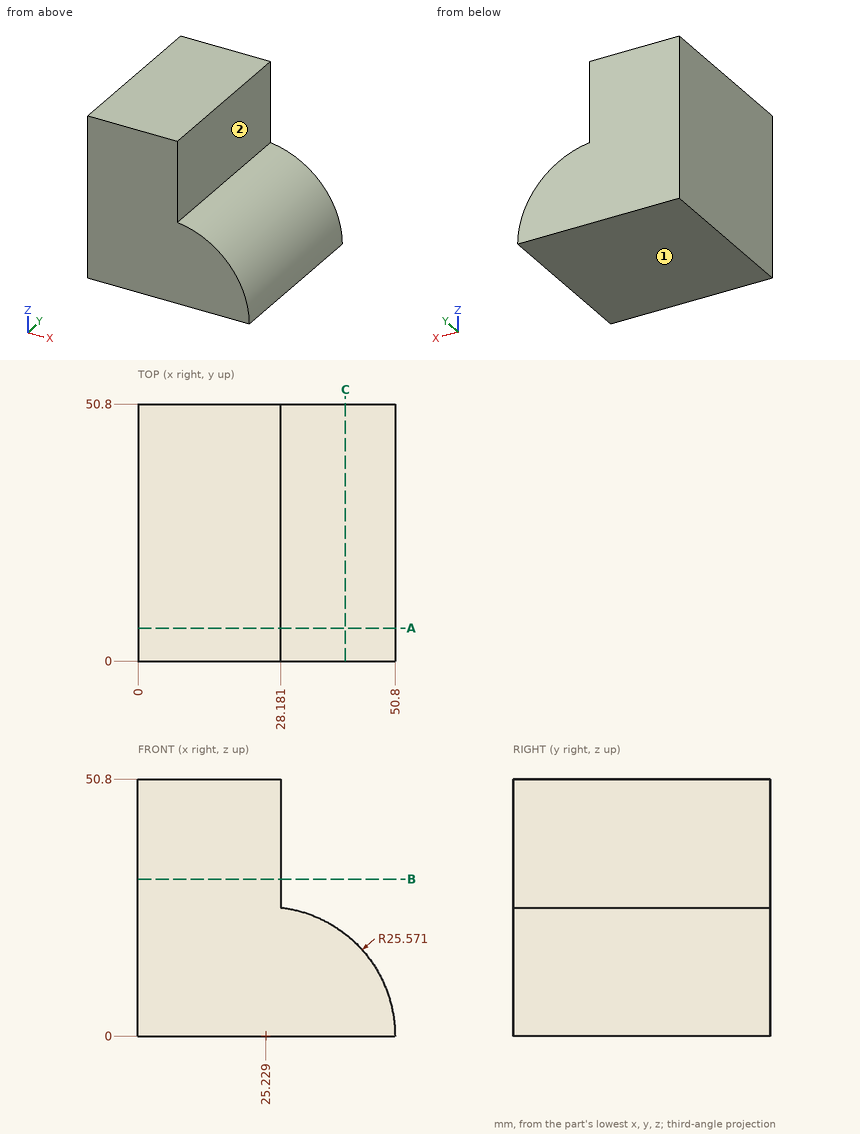
The drawing under review shows one solid part. Ordinate dimensions are in mm from its lowest x, y, z. A direction names the side the tool comes from. Round coordinates to 2 decimals unless told otherwise and drop trailing zeros. Write each loop counter-clockwise with the first axis right and the second up, starting at its lowest first coordinate (ties: lowest second). Pieces come first, ordered by that corner, then holes. Notation, with made-up numbers: M 87.5,40.5 L 105.5,40.5 A38 cw 105.5,79.5 Z; hole C 5.25,17 d4. An arc over 180 degrees is marked long. One line per item, written item: value. Start each with the question number.
(1) We need section B-B (z = 31). Give the boundary of the cut face in (x, y), and give its area (3 significant figures).
(2) Insertion check: pin 1 (2 mm diameter, centred on y = 37, z = 11.5, fed in from +X) (1 decimal); pin 2 (3 mm diameter, centred on y = 6.5, z = 42, fed in from +X); pin 3 (5 mm diameter, centred on x = 37, z = 26, fed in from -Y). Each pin has a flat end and moves straight along its axis. Give the tip position at first contact, or say it passes through.
(3) Machinability: for the marked faces 1 and 2, which of the approach directions +Z, -Z, +X, -X, +Y, -Y give a long, thin tool a straight path to every point of the face, cutting with its end or side? Answer none if there is none.
(4) We need section C-C (x = 41). Give the boundary of the cut face in (y, z).
(5) We need section A-A (y = 6.5). Give the boundary of the cut face in (x, z).
(6) Wall thickness on line 1 (X direction, y = 33.5, z = 37); line 2 (Z direction, x = 30, y = 35.5); line 3 (X direction, y = 43, z = 20) (1 decimal): over which ranges is each line inside the solid? List them lowest first.
Result:
1. outline: M 0,0 L 28.18,0 L 28.18,50.8 L 0,50.8 Z
1. area: 1,430 mm²
2. pin 1: x = 48.5
2. pin 2: x = 28.18
2. pin 3: through
3. face 1: -Z, +X, -X, +Y, -Y
3. face 2: +Z, +X, +Y, -Y
4. outline: M 0,0 L 50.8,0 L 50.8,20.13 L 0,20.13 Z
5. outline: M 0,0 L 50.8,0 A25.57 ccw 28.18,25.4 L 28.18,50.8 L 0,50.8 Z
6. line 1: 0 to 28.18
6. line 2: 0 to 25.12
6. line 3: 0 to 41.2
